```python
from build123d import *

# Parameters (mm, degrees)
SKETCH1_W           = 200
SKETCH1_H           = 150
BOSS_EXTRUDE1_DEPTH = 150
CUT_EXTRUDE1_DEPTH  = 235.520787991
SKETCH3_W           = 130
SKETCH3_H           = 130
CUT_EXTRUDE2_DEPTH  = 262.007662723
SKETCH4_R           = 60
CUT_EXTRUDE3_DEPTH  = 196.256241898
SKETCH5_R           = 71.933937191
BOSS_EXTRUDE2_DEPTH = 82


with BuildPart() as part:
    # Sketch1 → Boss-Extrude1 (new body)
    with BuildSketch(Plane(origin=(0, 0, 0), x_dir=(1, 0, 0), z_dir=(0, 1, 0))):
        Rectangle(SKETCH1_W, SKETCH1_H)
    extrude(amount=BOSS_EXTRUDE1_DEPTH)

    # Sketch2 → Cut-Extrude1 (cut, through all)
    with BuildSketch(Plane.XY.offset(75)):
        Polygon((0, 132.735026919), (-50, 46.132486541), (50, 46.132486541), align=None)
    extrude(amount=-CUT_EXTRUDE1_DEPTH, mode=Mode.SUBTRACT)

    # Sketch3 → Cut-Extrude2 (cut, through all)
    with BuildSketch(Plane(origin=(100, 0, 0), x_dir=(0, 0, -1), z_dir=(1, 0, 0))):
        with Locations((0, 75)):
            Rectangle(SKETCH3_W, SKETCH3_H)
    extrude(amount=-CUT_EXTRUDE2_DEPTH, mode=Mode.SUBTRACT)

    # Sketch4 → Cut-Extrude3 (cut, through all)
    with BuildSketch(Plane(origin=(0, 150, 0), x_dir=(1, 0, 0), z_dir=(0, 1, 0))):
        with Locations(Location((0, 0, 0), (0, 0, 270))):
            Circle(SKETCH4_R)
    extrude(amount=-CUT_EXTRUDE3_DEPTH, mode=Mode.SUBTRACT)

    # Sketch5 → Boss-Extrude2 (add)
    with BuildSketch(Plane(origin=(0, 150, 0), x_dir=(1, 0, 0), z_dir=(0, 1, 0))):
        with Locations(Location((0, 0, 0), (0, 0, 90))):
            Circle(SKETCH5_R)
    extrude(amount=BOSS_EXTRUDE2_DEPTH)


solid = part.part
```
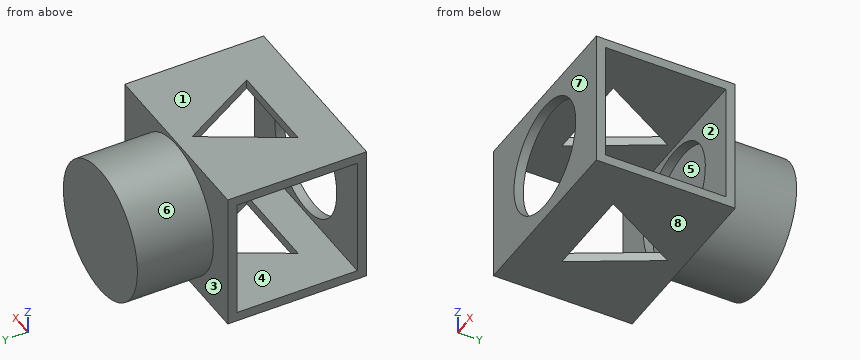
CAD build for the part. Positions are in the model's coordinates, mm. Face numbers are marked on the shaded views. A direction names the side the tool comes from. Round coordinates to 2 decimals unless told otherwise and drop trailing zeros. Loops run counter-clockwise (first coordinate to the right, second up) from the corner with the lowest first, then second, coordinate; pieces in that order, holes last. Notation, with made-up numbers: (81.25, -1.75) - (111.25, -1.75) arc R16 cw to (111.25, 13.25) - close; hole circle Ø7 at (-5, 71). An arc over 180 degrees is marked (long way). Return JSON: item names as keys, results as strings. Group by question number.
Q1. Two-plate mould, pull along Y, no slides. Class the marked faces 1, 2 and 3: +Y half, -Y half, draft (parallel to the pull), parting line (faces both ways), or undercut.
Q2. Tool access for the marked faces 4, 5, 6, 7 and 8: list every direction of +Z, -Z, +X, -X, +Y, -Y with a clear straight run to the whole face (end or side of a thin tool).
Q3. Drill centre lines: line 1 along X through (y, z) = (7, 0); line 2 along Y through (x, z) = (74.5, -52); line 3 along Y through (x, z) = (56, -34.5). Where is each one in solid material? Low to high. Write a range as [from, to].
Q4. Band-saw the part on A-A on x = -68.5. Give the cut face in (y, z), plus the area to 3 significant figures.
Q5. Band-saw the part on B-B on z = 0. Give the cut face in (x, y).
Q6. Flat gauge pin, fed straight in: pin 1 Ø4 at (x, z) = (71, -28.5) entering from +Y. Where does the tip first touch, or does it go through?
Q7. Band-saw the part on C-C on y = 38.5. Give the cut face in (x, z), plus the area to 3 significant figures.
Q8. Band-saw the part on D-D on x = 16.5. Give the cut face in (y, z), plus the area to 3 significant figures.
Solutions:
{
 "1": {"face 1": "draft", "face 2": "undercut", "face 3": "+Y half"},
 "2": {"face 4": "+X, -X", "face 5": "-Y", "face 6": "+Y", "face 7": "+Z, -Z, +X, -X, -Y", "face 8": "-Z, +X, -X, +Y, -Y"},
 "3": {"line 1": "x = [-100, -60], [60, 100]", "line 2": "y = [0, 10], [140, 150]", "line 3": "y = [0, 10], [140, 232]"},
 "4": {"outline": "(0, -75) - (150, -75) - (150, -21.96) - (232, -21.96) - (232, 21.96) - (150, 21.96) - (150, 75) - (0, 75) - close; hole (10, -65) - (140, -65) - (140, 65) - (10, 65) - close", "area": "9,200 mm^2"},
 "5": {"outline": "(-100, 0) - (-60, 0) - (-60, 10) - (-100, 10) - close; (-100, 140) - (-60, 140) - (-60, 150) - (60, 150) - (60, 140) - (100, 140) - (100, 150) - (71.93, 150) - (71.93, 232) - (-71.93, 232) - (-71.93, 150) - (-100, 150) - close; (60, 0) - (100, 0) - (100, 10) - (60, 10) - close"},
 "6": {"pin 1": "stops at y = 150"},
 "7": {"outline": "(-100, -75) - (100, -75) - (100, -65) - (-100, -65) - close; (-100, 65) - (100, 65) - (100, 75) - (-100, 75) - close", "area": "4,000 mm^2"},
 "8": {"outline": "(0, -75) - (46.13, -75) - (46.13, -65) - (10, -65) - (10, -57.69) - (0, -57.69) - close; (0, 57.69) - (10, 57.69) - (10, 65) - (46.13, 65) - (46.13, 75) - (0, 75) - close; (104.16, -75) - (150, -75) - (150, -70.02) - (232, -70.02) - (232, 70.02) - (150, 70.02) - (150, 75) - (104.16, 75) - (104.16, 65) - (140, 65) - (140, 57.69) - (150, 57.69) - (150, -57.69) - (140, -57.69) - (140, -65) - (104.16, -65) - close", "area": "13,600 mm^2"}
}
